```python
from build123d import *

# Parameters (mm, degrees)
SKETCH1_R           = 12.5
BOSS_EXTRUDE1_DEPTH = 40
BOSS_EXTRUDE2_DEPTH = 8
BOSS_EXTRUDE3_DEPTH = 80
SKETCH5_R           = 12.5
CUT_EXTRUDE1_DEPTH  = 96


with BuildPart() as part:
    # Sketch1 → Boss-Extrude1 (new, symmetric)
    with BuildSketch(Plane.XY):
        Circle(SKETCH1_R)
    extrude(amount=BOSS_EXTRUDE1_DEPTH, both=True)

    # Sketch2 → Boss-Extrude2 (add)
    with BuildSketch(Plane.XY.offset(40)):
        with BuildLine():
            Line((-19.868958458, 2.285714286), (-39.737916916, -170.428571429))
            ThreePointArc((-39.737916916, -170.428571429), (0, -215), (39.737916916, -170.428571429))
            Line((39.737916916, -170.428571429), (19.868958458, 2.285714286))
            ThreePointArc((19.868958458, 2.285714286), (0, 20), (-19.868958458, 2.285714286))
        make_face()
    boss_extrude2 = extrude(amount=BOSS_EXTRUDE2_DEPTH)

    # Mirror1: Boss-Extrude2 across plane
    add(boss_extrude2.mirror(Plane.XY))

    # Sketch4 → Boss-Extrude3 (add)
    with BuildSketch(Plane.XY.offset(-40)):
        with BuildLine():
            Line((-7.071067812, -121.645919803), (-35.177954833, -149.752806824))
            ThreePointArc((-35.177954833, -149.752806824), (-37.111501281, -152.47451583), (-38.04136625, -155.681017493))
            Line((-38.04136625, -155.681017493), (-39.737916916, -170.428571429))
            ThreePointArc((-39.737916916, -170.428571429), (0, -215), (39.737916916, -170.428571429))
            Line((39.737916916, -170.428571429), (38.04136625, -155.681017493))
            ThreePointArc((38.04136625, -155.681017493), (37.111501281, -152.47451583), (35.177954833, -149.752806824))
            Line((35.177954833, -149.752806824), (7.071067812, -121.645919803))
            ThreePointArc((7.071067812, -121.645919803), (0, -118.716987615), (-7.071067812, -121.645919803))
        make_face()
    extrude(amount=BOSS_EXTRUDE3_DEPTH)

    # Sketch5 → Cut-Extrude1 (cut)
    with BuildSketch(Plane(origin=(0, 0, -48), x_dir=(-1, 0, 0), z_dir=(0, 0, -1))):
        with Locations((0, -175)):
            Circle(SKETCH5_R)
    extrude(amount=-CUT_EXTRUDE1_DEPTH, mode=Mode.SUBTRACT)


solid = part.part
```
CAD build for the part. Positions are in the model's coordinates, mm. A direction names the side the tool comes from. Round coordinates to 2 decimals unless told otherwise and drop trailing zeros. Order: outer loops, then holes, each group sorted by start corner. A loop starts at its lowest first (then second) coordinate and runs counter-clockwise, first axis right, second up. Notation, with made-up numbers: (36.25, -10) - (63.25, -10) arc R16 cw to (63.25, 10) - close; hole circle Ø2 at (21, 33). An arc over 180 degrees is marked (long way). Use CSV: the item, a comma, the result in double quotes. Start each with the question number.
1) Wall check: L1, parallel to Y at x = 0, z = -11; L2, parallel to Y at x = 1, z = 1; L3, parallel to Z at x = 14, y = -117. Give the ranges that are in metal, low to high. Write a range as [from, to].
2) Saw through at D-D (x = -27.5). List the corners of the cut face in (y, z), and give its area (3 significant figures).
3) Saw through at A-A (z = -7.5). List the corners of the cut face in (x, y).
4) Two-plate mould, pull along Y, no slides. Class faces 5 (the cylindrical face through (-37.09, -152.43, -0.56)), 6 (the flat face through (-1, -96, 48)), 7 (the cylindrical face through (0.11, -118.718, -0.56)): pulls with the +Y half, pulls with the -Y half, needs draft (parallel to the pull), parting line crosses it, or undercut.
5) Tool access for faces 1 (the cylindrical face through (37.132, -152.517, -0.56)), 2 (the flat face through (21.321, -135.896, -0.56)), 3 (the cylindrical face through (11.923, 3.755, 0.56)), 4 (the flat face through (-20.928, -135.503, -0.56)): list every direction of +Z, -Z, +X, -X, +Y, -Y with a clear straight run to the whole face (end or side of a thin tool).
6) Saw through at C-C (x = 0). List the corners of the cut face in (y, z).
7) Saw through at B-B (y = -175). List the corners of the cut face in (x, z), and give its area (3 significant figures).
8) Pin check, flat tips, straight feed: pin 1 Ø1 at (y, z) = (-184, -11) entering from -X; pin 2 Ø8 at (y, z) = (-142.5, -21) entering from -X; pin 3 Ø1.5 at (x, z) = (15.5, 31) entering from -Y. Stop position of each tip, or through.
Values follow:
1,L1,"y = [-215, -187.5], [-162.5, -118.72], [-12.5, 12.5]"
1,L2,"y = [-214.99, -187.46], [-162.54, -118.77], [-12.46, 12.46]"
1,L3,"z = [-48, -40], [40, 48]"
2,outline,"(-204.05, -48) - (-64.05, -48) - (-64.05, -40) - (-142.07, -40) - (-142.07, 40) - (-64.05, 40) - (-64.05, 48) - (-204.05, 48) - close"
2,area,"7,200 mm2"
3,outline,"(-39.74, -170.43) arc R40 ccw (long way) to (39.74, -170.43) - (38.04, -155.68) arc R10 ccw to (35.18, -149.75) - (7.07, -121.65) arc R10 ccw to (-7.07, -121.65) - (-35.18, -149.75) arc R10 ccw to (-38.04, -155.68) - close; circle Ø25 at (0, 0); hole circle Ø25 at (0, -175)"
4,face 5,"pulls with the +Y half"
4,face 6,"needs draft"
4,face 7,"undercut"
5,face 1,"+X, +Y"
5,face 2,"+X"
5,face 3,"none"
5,face 4,"-X"
6,outline,"(-215, -48) - (-187.5, -48) - (-187.5, 48) - (-215, 48) - close; (-162.5, -48) - (20, -48) - (20, -40) - (12.5, -40) - (12.5, 40) - (20, 40) - (20, 48) - (-162.5, 48) - close; hole (-118.72, -40) - (-12.5, -40) - (-12.5, 40) - (-118.72, 40) - close"
7,outline,"(-40, -48) - (-12.5, -48) - (-12.5, 48) - (-40, 48) - close; (12.5, -48) - (40, -48) - (40, 48) - (12.5, 48) - close"
7,area,"5,280 mm2"
8,pin 1,"stops at x = -39.09"
8,pin 2,"stops at x = -31.93"
8,pin 3,"stops at y = -212.18"
